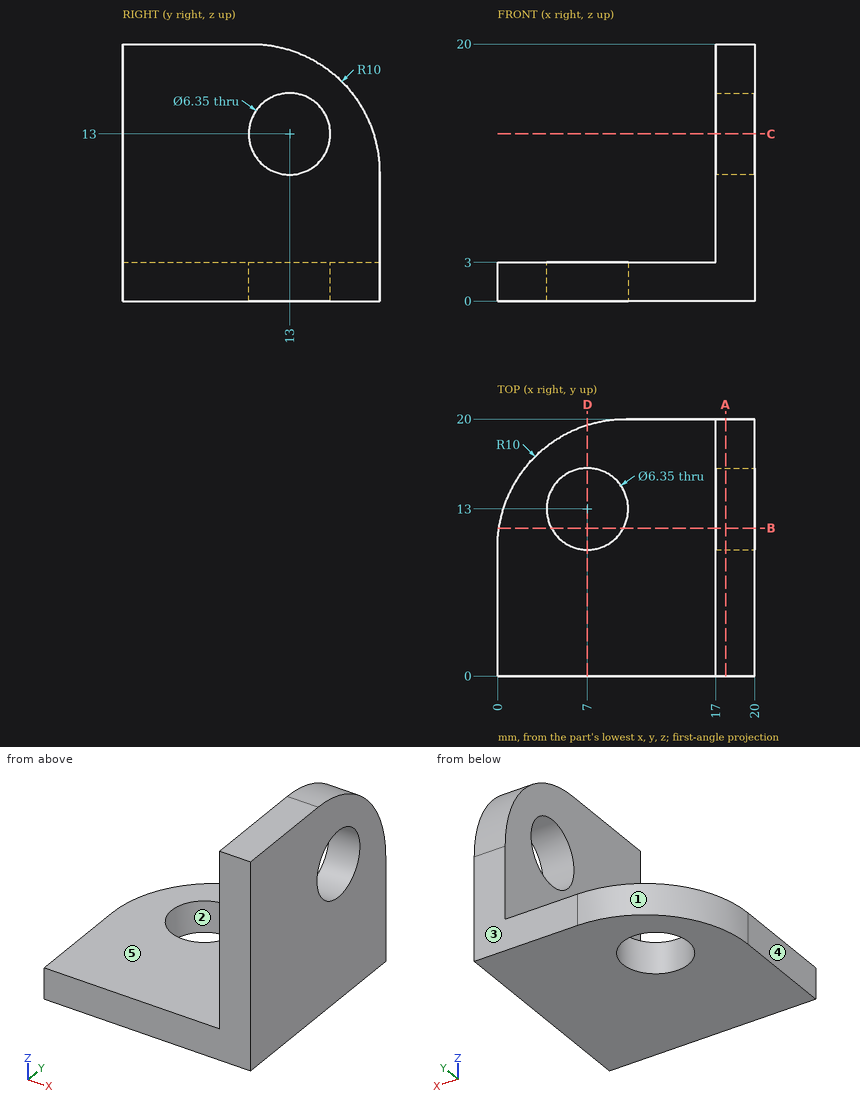
For this review, use the dimensioned drawing (mm, ordinates from the lowest corner) and the shaded views. A direction names the side the tool comes from. Round coordinates to 2 decimals unless told otherwise and drop trailing zeros. Order: outer loops, then holes, each group sorted by start corner. A loop starts at its lowest first (then second) coordinate and runs counter-clockwise, first axis right, second up. Notation, with made-up numbers: M 83.25,29 L 91.25,29 A30 cw 91.25,55 Z; hole C 53.25,74 d9. An arc over 180 degrees is marked long. Write each question's results on one line, items separated by ' | '. Start each with the question number.
1. Add section C-C (z = 13). State the section outline as (x, y) points (3 decimals), then the cut area to 3 significant figures.
2. Draft analysis for pull direction X (two halves, no side actions). For the marked faces 1, 2 and 3, state which applies: pulls with the +X half, pulls with the -X half, needs draft (parallel to the pull), parting line crosses it, or undercut.
3. Tool access review of the marked faces 4 and 5: name each direction out of +Z, -Z, +X, -X, +Y, -Y from which nothing blocks a thin tool from reaching the whole face with its end or side.
4. Clearance check with flat-ended pins moving along their axes: pin 1 Ø6 at (y, z) = (11.5, 7.5) entering from -X; pin 2 Ø2 at (x, y) = (4, 6.5) entering from +Z. State where each tip first meets the part, or that it passes through.
5. Add section D-D (x = 7). State the section outline as (y, z) points (3 decimals).
6. Add section A-A (x = 17.75). State the section outline as (y, z) points (3 decimals), then the cut area to 3 significant figures.
7. Add section B-B (y = 11.5). State the section outline as (x, z) points.
8. To check wall thickness, follow L1, parallel to Z at x = 5.5, y = 17.25; L2, parallel to X at y = 18.5, z = 7; L3, parallel to Y at x = 18.8, z = 13 (3 decimals). State the ranges of each line that lie inside material, in increasing order. Write a range as [from, to].
Output values:
1) outline: M 17,0 L 20,0 L 20,9.825 L 17,9.825 Z; M 17,16.175 L 20,16.175 L 20,19.539 L 17,19.539 Z | area: 39.6 mm^2
2) face 1: pulls with the -X half | face 2: undercut | face 3: needs draft
3) face 4: +Z, -Z, -X, +Y, -Y | face 5: +Z, -X, +Y, -Y
4) pin 1: x = 17 | pin 2: z = 3
5) outline: M 0,0 L 9.825,0 L 9.825,3 L 0,3 Z; M 16.175,0 L 19.539,0 L 19.539,3 L 16.175,3 Z
6) outline: M 0,0 L 20,0 L 20,10 A10 ccw 10,20 L 0,20 Z; hole C 13,13 d6.35 | area: 347 mm^2
7) outline: M 0.11,0 L 4.2,0 L 4.2,3 L 0.11,3 Z; M 9.8,0 L 20,0 L 20,10.2 L 17,10.2 L 17,3 L 9.8,3 Z; M 17,15.8 L 20,15.8 L 20,19.89 L 17,19.89 Z
8) L1: [0, 3] | L2: [17, 20] | L3: [0, 9.825], [16.175, 19.539]
